```python
from build123d import *

# Parameters (mm, degrees)
SKETCH1_R                     = 62.09
BOSS_EXTRUDE1_DEPTH           = 17
BOSS_EXTRUDE1_OTHER_WAY_DEPTH = 10
BOSS_EXTRUDE1_OTHER_WAY_TAPER = 70
SKETCH2_R                     = 43.87
BOSS_EXTRUDE2_DEPTH           = 15
BOSS_EXTRUDE2_TAPER           = 55
SKETCH3_R                     = 17.71
CUT_EXTRUDE1_DEPTH            = 98.336202069


with BuildPart() as part:
    # Sketch1 → Boss-Extrude1 (new body)
    with BuildSketch(Plane.XY):
        Circle(SKETCH1_R)
    extrude(amount=BOSS_EXTRUDE1_DEPTH)

    # Sketch1 → Boss-Extrude1 other way (add)
    with BuildSketch(Plane.XY):
        Circle(SKETCH1_R)
    extrude(amount=-BOSS_EXTRUDE1_OTHER_WAY_DEPTH, taper=BOSS_EXTRUDE1_OTHER_WAY_TAPER)

    # Sketch2 → Boss-Extrude2 (add)
    with BuildSketch(Plane.XY.offset(17)):
        Circle(SKETCH2_R)
    extrude(amount=BOSS_EXTRUDE2_DEPTH, taper=BOSS_EXTRUDE2_TAPER)

    # Sketch3 → Cut-Extrude1 (cut, through all)
    with BuildSketch(Plane.XY.offset(32)):
        Circle(SKETCH3_R)
    extrude(amount=-CUT_EXTRUDE1_DEPTH, mode=Mode.SUBTRACT)


solid = part.part
```
Geometry: final body of the model. Coordinates: model frame, mm. A direction names the side the tool comes from. Round coordinates to 2 decimals unless told otherwise and drop trailing zeros. Order: outer loops, then holes, each group sorted by start corner. A loop starts at its lowest first (then second) coordinate and runs counter-clockwise, first axis right, second up. Notation, with made-up numbers: (28.25, -4) -> (42.25, -4) arc R19 ccw to (42.25, 9) -> close; hole circle Ø6 at (68.5, 17). An arc over 180 degrees is marked (long way). Write each question's results on one line, items separated by ' | '.
Q1. Section query B-B (z = 6). Output: boundary loops of the cut face in (x, y).
Response values:
outline: circle Ø124.18 at (0, 0); hole circle Ø35.42 at (0, 0)
Q2. Pull-direction query (X, two-part tool) for faces 3 (the face through (-7.793, -35.094, -9.514)), 4 (the face through (-2.31, 17.56, 11.29)), 5 (the face through (-16, 8, -10)); classes: released by +X, released by -X, zero draft, split by the parting line, or undercut.
Response values:
face 3: split by the parting line | face 4: undercut | face 5: zero draft
Q3. Access query for faces 1 (the face through (12.9, 42.3, 17)), 2 (the face through (17, 7, 32)). Directions: +Z, -Z, +X, -X, +Y, -Y. A direction counts if a zero-diameter tool reaches every point of the face in a straight line with its end or side. Return the directions, or none.
Response values:
face 1: +Z | face 2: +Z, +X, -X, +Y, -Y
Q4. Section query A-A (x = 0). Output: boundary loops of the cut face in (y, z), and give its area (3 significant figures).
Response values:
outline: (-62.09, 0) -> (-34.62, -10) -> (-17.71, -10) -> (-17.71, 32) -> (-22.45, 32) -> (-43.87, 17) -> (-62.09, 17) -> close; (17.71, -10) -> (34.62, -10) -> (62.09, 0) -> (62.09, 17) -> (43.87, 17) -> (22.45, 32) -> (17.71, 32) -> close | area: 2,590 mm²
Q5. Ray query, line 1 along Y through (x, z) = (0, 2); line 2 along X through (y, z) = (10, 11.5); line 3 along Y through (x, z) = (12.5, 23). Return the intervals inside material, ascending.
Response values:
line 1: -62.09 to -17.71, 17.71 to 62.09 | line 2: -61.28 to -14.62, 14.62 to 61.28 | line 3: -33.01 to -12.55, 12.55 to 33.01
Q6. Pin query (flat end, axial travel): pin 1 Ø4 at (x, y) = (-7, -13.5) entering from +Z; pin 2 Ø10 at (x, y) = (3, 29) entering from +Z; pin 3 Ø12 at (x, z) = (-20, 18.5) entering from -Y; pin 4 Ø12 at (y, z) = (-32.5, -2) entering from +X. Return the tip coordinate at first contact, or that it passes through.
Response values:
pin 1: through | pin 2: z = 30.8 | pin 3: y = -60.45 | pin 4: x = 55.99
Q7. Section query C-C (z = 29). Output: boundary loops of the cut face in (x, y), and give its area (3 significant figures).
Response values:
outline: circle Ø53.46 at (0, 0); hole circle Ø35.42 at (0, 0) | area: 1,260 mm²
